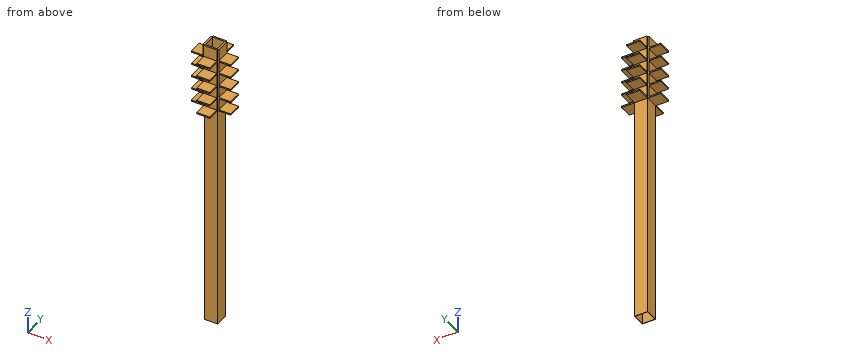
```python
from build123d import *

# Parameters (mm, degrees)
F0_W          = 31.75
F0_H          = 31.75
F0_W_2        = 30.1625
F0_H_2        = 30.1625
F1_DEPTH      = 711.2
F5_START      = 552.45
F4_W          = 31.75
F4_H          = 31.75
F5_DEPTH      = 158.75
F6_W          = 28.575
F6_H          = 28.575
F7_DEPTH      = 25.4
F7_DEPTH_BACK = 25.4
F8_W          = 28.575
F8_H          = 28.575
F9_DEPTH      = 25.4
F9_DEPTH_BACK = 25.4
F11_START     = 552.45
F10_W         = 30.1625
F10_H         = 30.1625
F11_DEPTH     = 158.75


with BuildPart() as f1:
    # F0 (on Top) → F1 (new body)
    with BuildSketch(Plane.XY):
        Rectangle(F0_W, F0_H)
        Rectangle(F0_W_2, F0_H_2, mode=Mode.SUBTRACT)
    extrude(amount=F1_DEPTH)

    # F4 (on Top) → F5 (join)
    with BuildSketch(Plane.XY.offset(F5_START)):
        with Locations((31.75, 0)):
            Rectangle(F4_W, F4_H)
        with Locations((-31.75, 0)):
            Rectangle(F4_W, F4_H)
        with Locations((0, 31.75)):
            Rectangle(F4_W, F4_H)
        with Locations((0, -31.75)):
            Rectangle(F4_W, F4_H)
    extrude(amount=F5_DEPTH)

    # F6 (on Front) → F7 (cut, two sides)
    with BuildSketch(Plane.XZ) as f7_sk:
        with Locations((33.3375, 665.1625)):
            Rectangle(F6_W, F6_H)
        with Locations((33.3375, 696.9125)):
            Rectangle(F6_W, F6_H)
        with Locations((-33.3375, 696.9125)):
            Rectangle(F6_W, F6_H)
        with Locations((-33.3375, 665.1625)):
            Rectangle(F6_W, F6_H)
        with Locations((33.3375, 633.4125)):
            Rectangle(F6_W, F6_H)
        with Locations((33.3375, 601.6625)):
            Rectangle(F6_W, F6_H)
        with Locations((33.3375, 569.9125)):
            Rectangle(F6_W, F6_H)
        with Locations((-33.3375, 633.4125)):
            Rectangle(F6_W, F6_H)
        with Locations((-33.3375, 601.6625)):
            Rectangle(F6_W, F6_H)
        with Locations((-33.3375, 569.9125)):
            Rectangle(F6_W, F6_H)
    extrude(amount=-F7_DEPTH, mode=Mode.SUBTRACT)
    extrude(f7_sk.sketch, amount=F7_DEPTH_BACK, mode=Mode.SUBTRACT)

    # F8 (on Right) → F9 (cut, two sides)
    with BuildSketch(Plane.YZ) as f9_sk:
        with Locations((33.3375, 696.9125)):
            Rectangle(F8_W, F8_H)
        with Locations((33.3375, 665.1625)):
            Rectangle(F8_W, F8_H)
        with Locations((-33.3375, 696.9125)):
            Rectangle(F8_W, F8_H)
        with Locations((-33.3375, 665.1625)):
            Rectangle(F8_W, F8_H)
        with Locations((33.3375, 633.4125)):
            Rectangle(F8_W, F8_H)
        with Locations((33.3375, 601.6625)):
            Rectangle(F8_W, F8_H)
        with Locations((33.3375, 569.9125)):
            Rectangle(F8_W, F8_H)
        with Locations((-33.3375, 633.4125)):
            Rectangle(F8_W, F8_H)
        with Locations((-33.3375, 601.6625)):
            Rectangle(F8_W, F8_H)
        with Locations((-33.3375, 569.9125)):
            Rectangle(F8_W, F8_H)
    extrude(amount=-F9_DEPTH, mode=Mode.SUBTRACT)
    extrude(f9_sk.sketch, amount=F9_DEPTH_BACK, mode=Mode.SUBTRACT)


with BuildPart() as f11:
    # F10 (on Top) → F11 (new body)
    with BuildSketch(Plane.XY.offset(F11_START)):
        Rectangle(F10_W, F10_H)
    extrude(amount=F11_DEPTH)


solid = f1.part
```
Verification items for the finished model (mm, model axes). Give positions to 0.01 mm unless a question says otherwise; leave off trailing zeros. Loops run counter-clockwise (first coordinate to the right, second up) from the corner with the lowest first, then second, coordinate; pieces in that order, holes last.
1. Go/stop test with flat-tipped pins: pin 1 Ø8.5 at (x, y) = (39.5, 4) entering from -Z; pin 2 Ø8.5 at (x, z) = (4.5, 695) entering from -Y; pin 3 Ø23 at (y, z) = (-5.5, 703) entering from -X. Record where each tip stops, or that it passes through.
2. Thickness scan on line 1 (Z direction, x = -10, y = 35.5) (3 decimals); line 2 (X direction, y = 13, z = 583.5); line 3 (X direction, y = -9, z = 67) (3 decimals). Record the ranges inside material, lowest first.
3. Section check A-A, the plane y = 36. Enter the section's corners in (x, z) (3 decimals).
4. Section check B-B, the plane z = 155. Enter the section's corners in (x, y) (3 decimals).
Geometry says:
1. pin 1: stops at z = 552.45
1. pin 2: stops at y = -19.05
1. pin 3: stops at x = -19.05
2. line 1: z = 552.45 to 555.625, 584.2 to 587.375, 615.95 to 619.125, 647.7 to 650.875, 679.45 to 682.625
2. line 2: x = -19.05 to -15.08, 15.08 to 19.05
2. line 3: x = -15.875 to -15.081, 15.081 to 15.875
3. outline: (-15.875, 552.45) - (15.875, 552.45) - (15.875, 555.625) - (-15.875, 555.625) - close; (-15.875, 584.2) - (15.875, 584.2) - (15.875, 587.375) - (-15.875, 587.375) - close; (-15.875, 615.95) - (15.875, 615.95) - (15.875, 619.125) - (-15.875, 619.125) - close; (-15.875, 647.7) - (15.875, 647.7) - (15.875, 650.875) - (-15.875, 650.875) - close; (-15.875, 679.45) - (15.875, 679.45) - (15.875, 682.625) - (-15.875, 682.625) - close
4. outline: (-15.875, -15.875) - (15.875, -15.875) - (15.875, 15.875) - (-15.875, 15.875) - close; hole (-15.081, -15.081) - (15.081, -15.081) - (15.081, 15.081) - (-15.081, 15.081) - close
